Input: part model. Units: mm. Frame: model coordinates. Face numbers are marked on the shaded views. A direction names the side the tool comes from. Coordinates: 2 decimals unless noted, no trailing zeros. Loops run counter-clockwise (first coordinate to the right, second up) from the corner with the lowest first, then second, coordinate; pieces in that order, holes last.
Item 1: Ray query, line 1 along Z through (x, y) = (10, 1); line 2 along Z through (x, y) = (-10, 1.1); line 3 along X through (y, z) = (5, -3). Return the intervals inside material, ascending.
Item 2: Section D-D on x = 17. Return loops of the section in (y, z).
Item 3: Section A-A on z = 10. Return loops of the section in (x, y), and give its area (4 significant figures).
Item 4: Reachability of the marked faces 1, 2, 3 and 4 from +Z, -Z, +X, -X, +Y, -Y: full face, straight path, thin tool, end or side. Return the list, or none.
Item 5: Section B-B on x = -10. Return loops of the section in (y, z), and give its area (4 significant figures).
Item 6: Section C-C on y = 1. Return loops of the section in (x, z), and give its area (3 significant figures).
Item 7: Contact query for flat-ended pins moving along their axis: P1, Ø1.2, axis at y = 1, z = 0.5, coming from the -X side; P2, Ø1.6, axis at y = 5, z = 1, coming from the +X side; P3, Ø2.5, axis at y = 4.5, z = 14, coming from the -X side. Output: stop coordinate, or through.
```python
from build123d import *

# Parameters (mm, degrees)
SKETCH1_W           = 40
SKETCH1_H           = 40
BOSS_EXTRUDE1_DEPTH = 1.5
SKETCH2_R           = 1.5
BOSS_EXTRUDE2_DEPTH = 1.5
SKETCH3_R           = 1
SKETCH3_R_2         = 2.5
CUT_EXTRUDE1_DEPTH  = 1.5
SKETCH4_W           = 8
SKETCH4_H           = 12
BOSS_EXTRUDE3_DEPTH = 5.5
SKETCH5_W           = 27
SKETCH5_H           = 30
BOSS_EXTRUDE4_DEPTH = 7
SKETCH6_W           = 11
SKETCH6_H           = 3
BOSS_EXTRUDE5_DEPTH = 6.5
FILLET1_R           = 2


with BuildPart() as part:
    # Sketch1 → Boss-Extrude1 (new body)
    with BuildSketch(Plane(origin=(0, 0, 0), x_dir=(1, 0, 0), z_dir=(0, 1, 0))):
        Rectangle(SKETCH1_W, SKETCH1_H)
    extrude(amount=BOSS_EXTRUDE1_DEPTH)

    # Sketch2 → Boss-Extrude2 (add)
    with BuildSketch(Plane(origin=(0, 1.5, 0), x_dir=(1, 0, 0), z_dir=(0, 1, 0))):
        with Locations((-20, 10)):
            Circle(SKETCH2_R)
        with Locations((10, 20)):
            Circle(SKETCH2_R)
        with Locations((20, -10)):
            Circle(SKETCH2_R)
        with Locations((-10, -20)):
            Circle(SKETCH2_R)
    extrude(amount=-BOSS_EXTRUDE2_DEPTH)

    # Sketch3 → Cut-Extrude1 (cut)
    with BuildSketch(Plane(origin=(0, 1.5, 0), x_dir=(1, 0, 0), z_dir=(0, 1, 0))):
        with Locations((-20, 10)):
            Circle(SKETCH3_R)
        with Locations((10, 20)):
            Circle(SKETCH3_R)
        with Locations((20, -10)):
            Circle(SKETCH3_R)
        with Locations((-10, -20)):
            Circle(SKETCH3_R)
        with Locations((-10, 20)):
            Circle(SKETCH3_R_2)
        with Locations((20, 10)):
            Circle(SKETCH3_R_2)
        with Locations((10, -20)):
            Circle(SKETCH3_R_2)
        with Locations((-20, -10)):
            Circle(SKETCH3_R_2)
    extrude(amount=-CUT_EXTRUDE1_DEPTH, mode=Mode.SUBTRACT)

    # Sketch4 → Boss-Extrude3 (add)
    with BuildSketch(Plane(origin=(0, 1.5, 0), x_dir=(1, 0, 0), z_dir=(0, 1, 0))):
        with Locations((-13.43888983, 0)):
            Rectangle(SKETCH4_W, SKETCH4_H)
    extrude(amount=BOSS_EXTRUDE3_DEPTH)

    # Sketch5 → Boss-Extrude4 (add)
    with BuildSketch(Plane(origin=(0, 1.5, 0), x_dir=(1, 0, 0), z_dir=(0, 1, 0))):
        with Locations((4.5, 2)):
            Rectangle(SKETCH5_W, SKETCH5_H)
    extrude(amount=BOSS_EXTRUDE4_DEPTH)

    # Sketch6 → Boss-Extrude5 (add)
    with BuildSketch(Plane(origin=(0, 1.5, 0), x_dir=(1, 0, 0), z_dir=(0, 1, 0))):
        with Locations((4.5, -14.5)):
            Rectangle(SKETCH6_W, SKETCH6_H)
    extrude(amount=BOSS_EXTRUDE5_DEPTH)

    # Fillet1
    fillet1_edges = [part.edges().sort_by_distance(p)[0] for p in [
        (4.5, 8, 16),
    ]]
    fillet(fillet1_edges, radius=FILLET1_R)


solid = part.part
```
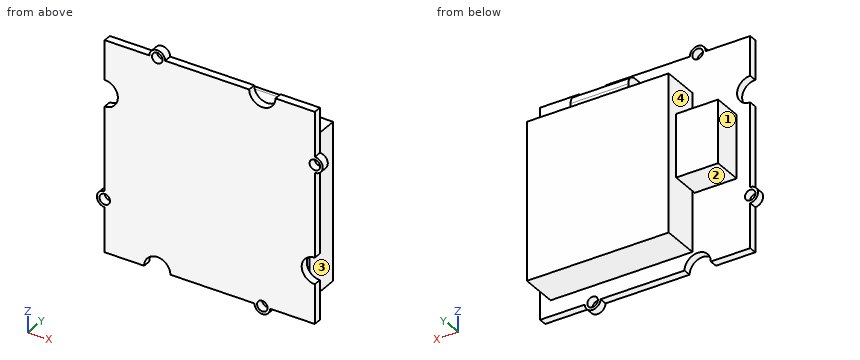
Results found:
1. line 1: z = -21.5 to -21, -19 to 17.5
1. line 2: z = -17.5 to 19, 21 to 21.5
1. line 3: x = -17.44 to -9.44, -9 to 18
2. outline: (0, -20) - (1.5, -20) - (1.5, -17) - (8.5, -17) - (8.5, 13) - (1.5, 13) - (1.5, 20) - (0, 20) - close
3. outline: (-17.5, 0) - (19, 0) - (19, 1.5) - (18, 1.5) - (18, 8.5) - (-9, 8.5) - (-9, 1.5) - (-17.5, 1.5) - close; (21, 0) - (21.5, 0) - (21.5, 1.5) - (21, 1.5) - close
3. area: 244.5 mm2
4. face 1: +Z, -Z, -X, +Y
4. face 2: -Z, -X, +Y
4. face 3: +Z, -Z, +X, +Y
4. face 4: +Z, -Z, +Y
5. outline: (0, -17.5) - (1.5, -17.5) - (1.5, -6) - (7, -6) - (7, 6) - (1.5, 6) - (1.5, 19) - (0, 19) - close; (0, 21) - (1.5, 21) - (1.5, 21.5) - (0, 21.5) - close
5. area: 121.5 mm2
6. outline: (-20, -20) - (-12.5, -20) arc R2.5 cw to (-7.5, -20) - (8.5, -20) arc R1.5 ccw to (11.5, -20) - (20, -20) - (20, -12.5) arc R2.5 cw to (20, -7.5) - (20, 8.5) arc R1.5 ccw to (20, 11.5) - (20, 20) - (12.5, 20) arc R2.5 cw to (7.5, 20) - (-8.5, 20) arc R1.5 ccw to (-11.5, 20) - (-20, 20) - (-20, 12.5) arc R2.5 cw to (-20, 7.5) - (-20, -8.5) arc R1.5 ccw to (-20, -11.5) - close; hole circle Ø2 at (-20, -10); hole circle Ø2 at (-10, 20); hole circle Ø2 at (10, -20); hole circle Ø2 at (20, 10)
6. area: 1,560 mm2
7. P1: stops at x = -20
7. P2: stops at x = 18
7. P3: stops at x = -9
